Geometry: see drawing. Coordinates: mm, zero at the bounding-box minimum. A direction names the side the tool comes from. Round coordinates to 2 decimals unless told otherwise and drop trailing zeros. Write each loop counter-clockwise with the first axis right and the second up, starting at its lowest first coordinate (ties: lowest second). Pieces come first, ordered by that corner, then holes.
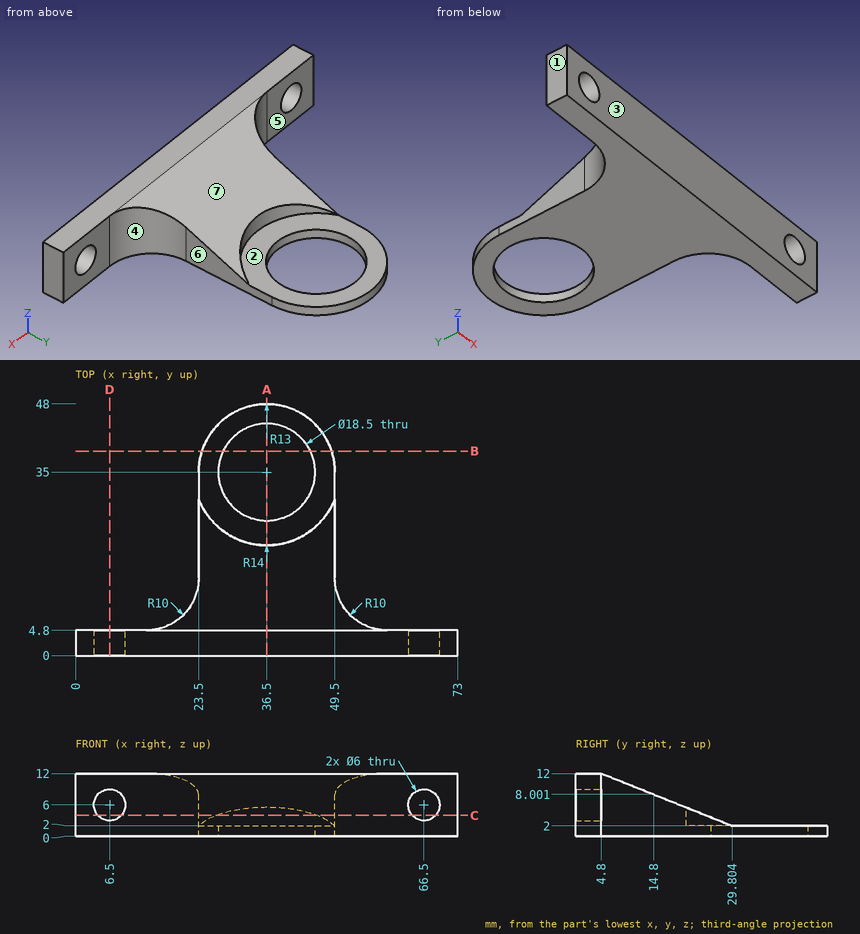
1) Material intervals for line 1 (Y direction, x = 36.5, z = 1.05); line 2 (Z direction, x = 6.5, y = 2.55); line 3 (Y direction, x = 12.5, z = 4), sorted ascending.
Taken from the geometry:
line 1: y = 0 to 25.75, 44.25 to 48
line 2: z = 0 to 3, 9 to 12
line 3: y = 0 to 4.8
2) Section query A-A on x = 36.5. Return the cut outline in (y, z).
Taken from the geometry:
outline: (0, 0) - (25.75, 0) - (25.75, 2) - (21, 2) - (21, 5.52) - (4.8, 12) - (0, 12) - close; (44.25, 0) - (48, 0) - (48, 2) - (44.25, 2) - close
3) Reachability of the marked faces 5, 6 and 7 from +Z, -Z, +X, -X, +Y, -Y: full face, straight path, thin tool, end or side. Return the list, or none.
Taken from the geometry:
face 5: +Z, -Z, -X, +Y
face 6: +Z, -Z, +X, +Y
face 7: +Z, +X, -X, +Y
4) Section query D-D on x = 6.5. Return the cut outline in (y, z).
Taken from the geometry:
outline: (0, 0) - (4.8, 0) - (4.8, 3) - (0, 3) - close; (0, 9) - (4.8, 9) - (4.8, 12) - (0, 12) - close
5) Pull-direction query (X, two-part tool) for the marked faces 1, 2, 3 and 4; classes: released by +X, released by -X, zero draft, split by the parting line, or undercut.
Taken from the geometry:
face 1: released by -X
face 2: undercut
face 3: zero draft
face 4: released by +X
6) Section query C-C on z = 4. Return the cut outline in (x, y).
Taken from the geometry:
outline: (0, 0) - (4.26, 0) - (4.26, 4.8) - (0, 4.8) - close; (8.74, 0) - (64.26, 0) - (64.26, 4.8) - (59.5, 4.8) arc R10 cw to (49.5, 14.8) - (49.5, 24.8) - (46.09, 24.8) arc R14 cw to (26.91, 24.8) - (23.5, 24.8) - (23.5, 14.8) arc R10 cw to (13.5, 4.8) - (8.74, 4.8) - close; (68.74, 0) - (73, 0) - (73, 4.8) - (68.74, 4.8) - close
7) Section query B-B on y = 39. Return the cut outline in (x, z), then the cut area to 3 significant figures.
Taken from the geometry:
outline: (24.13, 0) - (28.16, 0) - (28.16, 2) - (24.13, 2) - close; (44.84, 0) - (48.87, 0) - (48.87, 2) - (44.84, 2) - close
area: 16.1 mm2
8) Contact query for flat-ended pins moving along their axis: P1, Ø16.5, axis at x = 36.5, y = 35, coming from the -Z side; P2, Ø3, axis at x = 50.5, y = 25.5, coming from the +Z side; P3, Ø6.5, axis at y = 21, z = 2.5, coming from the -X side; P4, Ø21, axis at x = 39, y = 34, coming from the +Z side. Output: stop coordinate, or through.
Taken from the geometry:
P1: passes through
P2: stops at z = 4.17
P3: stops at x = 23.5
P4: stops at z = 2
